Print and shaded views of the part. All mm, measured from the part's lowest x, y and z. A direction names the side the tool comes from. Coordinates: 2 decimals unless noted, no trailing zeros. Order: outer loops, then holes, each group sorted by start corner. A loop starts at its lowest first (then second) coordinate and runs counter-clockwise, first axis right, second up.
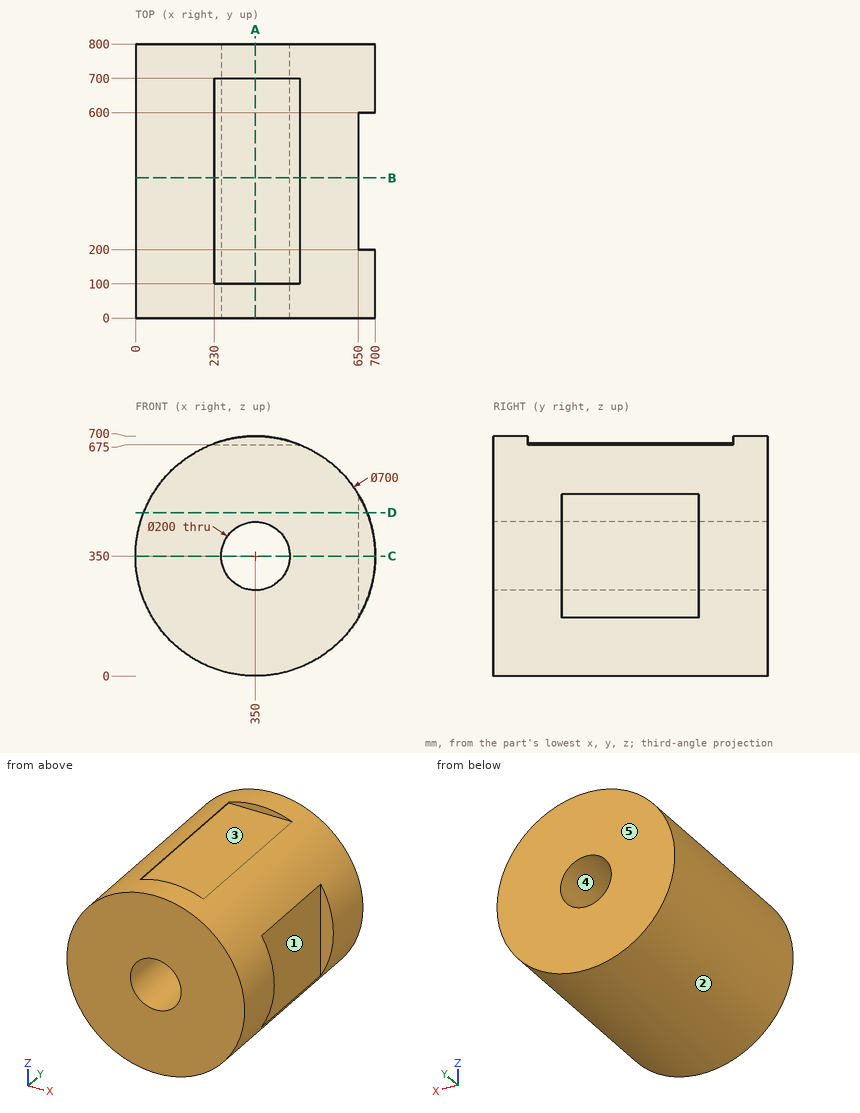
Q1. Probe line 1 (X direction, y = 319, z = 350); line 2 (X direction, y = 162, z = 350); line 3 (Z direction, x = 350, y = 280.5). List the from-to ranges inside material, lowest first.
Established:
line 1: x = 0 to 250, 450 to 650
line 2: x = 0 to 250, 450 to 700
line 3: z = 0 to 250, 450 to 675
Q2. Cut at C-C, the plane z = 350. List the corners of the cut face in (x, y).
Established:
outline: (0, 0) - (250, 0) - (250, 800) - (0, 800) - close; (450, 0) - (700, 0) - (700, 200) - (650, 200) - (650, 600) - (700, 600) - (700, 800) - (450, 800) - close
Q3. Drop flat-ended pins along their axis: P1, Ø1.5, axis at y = 339.5, z = 547.5, coming from the -X side; P2, Ø4, axis at y = 302.5, z = 204.5, coming from the +X side; P3, Ø1, axis at x = 423.5, y = 515.5, coming from the +Z side. Give the stop position or say it passes through.
Established:
P1: stops at x = 60.54
P2: stops at x = 650
P3: stops at z = 675
Q4. Which spindle directions (+Z, -Z, +X, -X, +Y, -Y) get a long thin tool onto all of the face, cutting with end or side? Do the marked faces 1 and 2. Say none if no direction does.
Established:
face 1: +Z, -Z, +X
face 2: +Y, -Y
Q5. Cut at D-D, the plane z = 477. List the corners of the cut face in (x, y).
Established:
outline: (23.85, 0) - (676.15, 0) - (676.15, 200) - (650, 200) - (650, 600) - (676.15, 600) - (676.15, 800) - (23.85, 800) - close
Q6. Cut at B-B, the plane y = 409. List the corners of the cut face in (x, z).
Established:
outline: (230, 675) - (230, 678.79) arc R350 ccw (long way) to (650, 169.72) - (650, 530.28) arc R350 ccw to (479.9, 675) - close; hole circle Ø200 at (350, 350)
Q7. Mould opens along Y. For the marked faces 3, 4 and 5 say: pulls with the +Y half, pulls with the -Y half, needs draft (parallel to the pull), parting line crosses it, or undercut.
Established:
face 3: undercut
face 4: needs draft
face 5: pulls with the +Y half
Q8. Cut at A-A, the plane x = 350. List the corners of the cut face in (y, z).
Established:
outline: (0, 0) - (800, 0) - (800, 250) - (0, 250) - close; (0, 450) - (800, 450) - (800, 700) - (700, 700) - (700, 675) - (100, 675) - (100, 700) - (0, 700) - close
